Answer from the drawing. Dimensions are ordinates in mm from the lowest x, y and z of the part. Round coordinates to 2 decimals unless told otherwise and drop trailing zeros. Loops run counter-clockwise (first coordinate to the right, second up) from the corner with the lowest first, then second, coordinate; pieces in that order, holes last. Notation, with made-up numbers: M 51,22 L 63,22 A30 cw 63,44 Z; hole C -8.75,86.5 d6. An arc over 180 degrees is marked long. Answer as a JSON object with one key per item and string values.
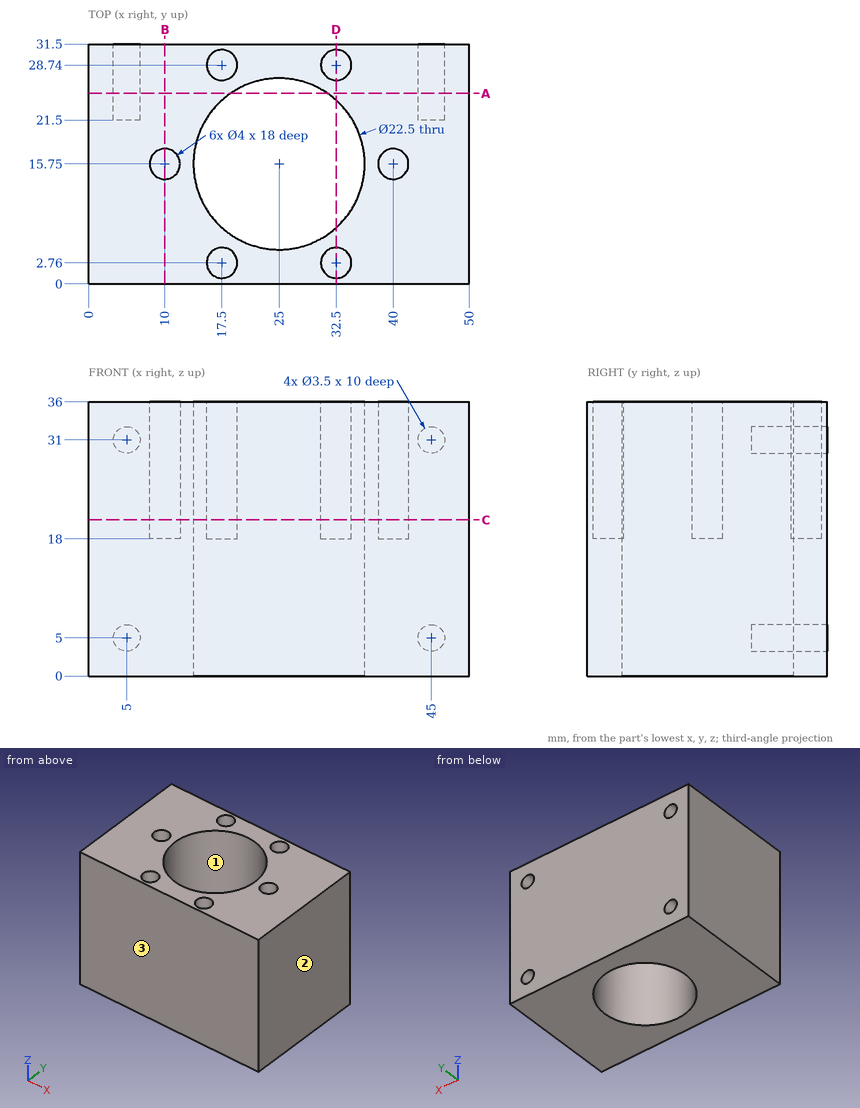
Item 1: The part is cut by section D-D (x = 32.5). Give the vertices of the cut face in (y, z) (1 decimal), then the cut area to 3 significant figures.
Values follow:
{"outline": "M 0,0 L 7.4,0 L 7.4,36 L 4.8,36 L 4.8,18 L 0.8,18 L 0.8,36 L 0,36 Z; M 24.1,0 L 31.5,0 L 31.5,36 L 30.7,36 L 30.7,18 L 26.7,18 L 26.7,36 L 24.1,36 Z", "area": "386 mm^2"}
Item 2: Determine the mould class of the marked faces 1, 2 and 3 for opening direction Y: released by +Y, released by -Y, zero draft, split by the parting line, or undercut.
Values follow:
{"face 1": "undercut", "face 2": "zero draft", "face 3": "released by -Y"}
Item 3: The part is cut by section A-A (y = 25). Give the vertices of the cut face in (x, z), then the cut area to 3 significant figures.
Values follow:
{"outline": "M 0,0 L 18.6,0 L 18.6,36 L 0,36 Z; M 31.4,0 L 50,0 L 50,36 L 31.4,36 Z; hole C 5,5 d3.5; hole C 5,31 d3.5; hole C 45,5 d3.5; hole C 45,31 d3.5", "area": "1,300 mm^2"}
Item 4: Straight lines are drawn through the part: line 1 (Y direction, x = 10, z = 28.5); line 2 (Y direction, x = 32.5, z = 25) (1 decimal); line 3 (Z direction, x = 4, y = 24) (1 decimal). For each, find the intervals that lie inside material, in ascending order.
Values follow:
{"line 1": "0 to 13.75, 17.75 to 31.5", "line 2": "0 to 0.8, 4.8 to 7.4, 24.1 to 26.7, 30.7 to 31.5", "line 3": "0 to 3.6, 6.4 to 29.6, 32.4 to 36"}
Item 5: The part is cut by section B-B (x = 10). Give the vertices of the cut face in (y, z).
Values follow:
{"outline": "M 0,0 L 31.5,0 L 31.5,36 L 17.75,36 L 17.75,18 L 13.75,18 L 13.75,36 L 0,36 Z"}
Item 6: Flat-ended cylindrical pins translate along their axes: P1, Ø2, axis at x = 5, z = 5, coming from the -Y side; P2, Ø1, axis at x = 4.5, z = 6, coming from the +Y side; P3, Ø13.5, axis at x = 25, y = 15.75, coming from the +Z side (3 decimals); P4, Ø1.2, axis at x = 17, y = 3.5, coming from the +Z side. Find the tip coordinate at first contact, or state that the pin passes through.
Values follow:
{"P1": "y = 0", "P2": "y = 21.5", "P3": "through", "P4": "z = 18"}
Item 7: The part is cut by section C-C (z = 20.5). Give the vertices of the cut face in (x, y).
Values follow:
{"outline": "M 0,0 L 50,0 L 50,31.5 L 0,31.5 Z; hole C 10,15.75 d4; hole C 25,15.75 d22.5; hole C 17.5,2.76 d4; hole C 17.5,28.74 d4; hole C 32.5,2.76 d4; hole C 32.5,28.74 d4; hole C 40,15.75 d4"}
